Could you check a few things on this model? Use its own coordinates, in mm. Face numbers are marked on the shaded views. A direction names the side the tool comes from. Coordinates: 2 decimals unless noted, no trailing zeros. Order: outer loops, then holes, each group sorted by start corner. A loop starts at its lowest first (then second) coordinate and runs counter-clockwise, first axis right, second up.
```python
from build123d import *

# Parameters (mm, degrees)
SKETCH1_W                = 15
SKETCH1_H                = 20
SKETCH1_R                = 2.51
BOSS_EXTRUDE1_DEPTH      = 3
SKETCH2_R                = 4.51
CUT_EXTRUDE1_DEPTH       = 1
BOSS_EXTRUDE2_DEPTH      = 22
BOSS_EXTRUDE2_DEPTH_BACK = 3
SKETCH3_W                = 3
SKETCH3_H                = 20
SKETCH4_R                = 2.6
CUT_EXTRUDE2_DEPTH       = 22
BOSS_EXTRUDE3_START      = -3
SKETCH5_R                = 2.6
BOSS_EXTRUDE3_DEPTH      = 3
CUT_EXTRUDE3_DEPTH       = 5
SKETCH7_W                = 20
SKETCH7_H                = 20
BOSS_EXTRUDE4_DEPTH      = 3
SKETCH8_R                = 2.6
CUT_EXTRUDE6_DEPTH       = 3


with BuildPart() as part:
    # Sketch1 → Boss-Extrude1 (new body)
    with BuildSketch(Plane(origin=(0, 0, 0), x_dir=(1, 0, 0), z_dir=(0, 1, 0))):
        with Locations((23.125880705, 19.115097078)):
            Rectangle(SKETCH1_W, SKETCH1_H)
        with Locations(Location((23.125880705, 19.115097078, 0), (0, 0, 270))):
            Circle(SKETCH1_R, mode=Mode.SUBTRACT)
    extrude(amount=BOSS_EXTRUDE1_DEPTH)

    # Sketch2 → Cut-Extrude1 (cut)
    with BuildSketch(Plane(origin=(0, 3, 0), x_dir=(1, 0, 0), z_dir=(0, 1, 0))):
        with Locations(Location((23.125880705, 19.115097078, 0), (0, 0, 270))):
            Circle(SKETCH2_R)
    extrude(amount=-CUT_EXTRUDE1_DEPTH, mode=Mode.SUBTRACT)

    # Sketch3 → Boss-Extrude2 (add, two sides: drawn at the far end of the back side and taken through both)
    with BuildSketch(Plane(origin=(0, 3, 0), x_dir=(1, 0, 0), z_dir=(0, 1, 0)).offset(-BOSS_EXTRUDE2_DEPTH_BACK)):
        with Locations((14.125880705, 19.115097078)):
            Rectangle(SKETCH3_W, SKETCH3_H)
    extrude(amount=BOSS_EXTRUDE2_DEPTH + BOSS_EXTRUDE2_DEPTH_BACK)

    # Sketch4 → Cut-Extrude2 (cut)
    with BuildSketch(Plane.ZY.offset(-12.625880705)):
        with Locations((-23.115097078, 19)):
            Circle(SKETCH4_R)
        with Locations((-23.115097078, 6)):
            Circle(SKETCH4_R)
    extrude(amount=-CUT_EXTRUDE2_DEPTH, mode=Mode.SUBTRACT)

    # Sketch5 → Boss-Extrude3 (add)
    with BuildSketch(Plane(origin=(15.625880705, 0, 0), x_dir=(0, 0, -1), z_dir=(1, 0, 0)).offset(BOSS_EXTRUDE3_START)):
        with Locations((23.115097078, 19)):
            Circle(SKETCH5_R)
        with Locations((23.115097078, 6)):
            Circle(SKETCH5_R)
    extrude(amount=BOSS_EXTRUDE3_DEPTH)

    # Sketch6 → Cut-Extrude3 (cut)
    with BuildSketch(Plane(origin=(12.625880705, 25, -29.115097078), x_dir=(1, 0, 0), z_dir=(0, 1, 0))):
        Polygon((0, -14.855128206), (0, -20), (3, -20), (3, -14.855128206), (3, 0), (0, 0), align=None)
    extrude(amount=-CUT_EXTRUDE3_DEPTH, mode=Mode.SUBTRACT)

    # Sketch7 → Boss-Extrude4 (add)
    with BuildSketch(Plane.ZY.offset(-12.625880705)):
        with Locations((-19.115097078, 30)):
            Rectangle(SKETCH7_W, SKETCH7_H)
    extrude(amount=-BOSS_EXTRUDE4_DEPTH)

    # Sketch8 → Cut-Extrude6 (cut)
    with BuildSketch(Plane(origin=(15.625880705, 0, 0), x_dir=(0, 0, -1), z_dir=(1, 0, 0))):
        with Locations((13.915097078, 16)):
            Circle(SKETCH8_R)
        with Locations((13.915097078, 26.1)):
            Circle(SKETCH8_R)
    extrude(amount=-CUT_EXTRUDE6_DEPTH, mode=Mode.SUBTRACT)


solid = part.part
```
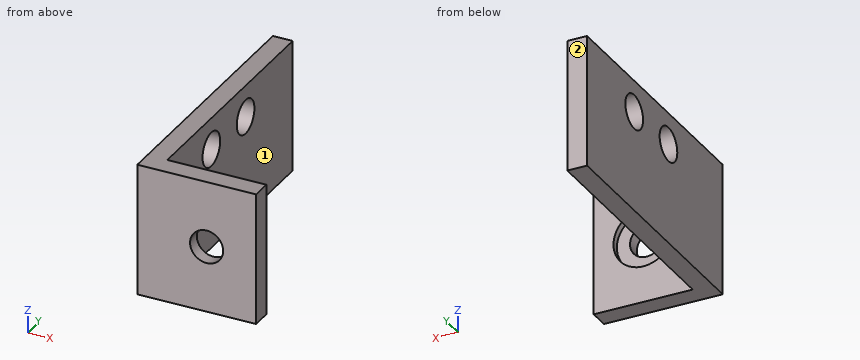
Item 1: I need wall thicknesses on line 1 (X direction, y = 11, z = -19); line 2 (Y direction, x = 21.75, z = -26); line 3 (Y direction, x = 24.5, z = -22.5). Which ranges of each line are inside material? Lowest first, please.
Item 2: Suppose I cut it at D-D (x = 22.25). List the corners of the cut face in (y, z) for me.
Item 3: Suppose I cut it at C-C (z = -13). List the corners of the cut face in (x, y) for me, and give its area (3 significant figures).
Item 4: For pin 1 Ø1 at (y, z) = (32.5, -17.5) entering from +X; pin 2 Ø4.5 at (y, z) = (16, -13.92) entering from -X; pin 3 Ø2 at (x, z) = (20, -14) entering from -Y; pin 4 Ø1 at (x, z) = (21, -19.5) entering from +Y, each with a flat end and sliding along its axis, tell me the tip position at first contact or that it passes through.
Item 5: Which directions (+Z, -Z, +X, -X, +Y, -Y) give clear straight access to the entire face, cutting with the end or side of a thin tool? Please do the marked faces 1 and 2.
Item 6: Suppose I cut it at A-A (y = 26.1). List the corners of the cut face in (x, z) for me.
Item 7: Suppose I cut it at B-B (x = 14.75). List the corners of the cut face in (y, z) for me, and give its area (3 significant figures).
Geometry results:
1. line 1: x = 12.63 to 15.63
1. line 2: y = 0 to 3
1. line 3: y = 0 to 2
2. outline: (0, -29.12) - (3, -29.12) - (3, -23.54) - (2, -23.54) - (2, -21.47) - (0, -21.47) - close; (0, -16.76) - (2, -16.76) - (2, -14.69) - (3, -14.69) - (3, -9.12) - (0, -9.12) - close
3. outline: (12.63, 0) - (30.63, 0) - (30.63, 3) - (15.63, 3) - (15.63, 13.57) - (12.63, 13.57) - close; (12.63, 18.43) - (15.63, 18.43) - (15.63, 23.67) - (12.63, 23.67) - close; (12.63, 28.53) - (15.63, 28.53) - (15.63, 40) - (12.63, 40) - close
3. area: 136 mm2
4. pin 1: stops at x = 15.63
4. pin 2: passes through
4. pin 3: stops at y = 0
4. pin 4: stops at y = 2
5. face 1: +Z, -Z, +X, +Y
5. face 2: +Z, -Z, +X, -X, +Y
6. outline: (12.63, -29.12) - (15.63, -29.12) - (15.63, -16.52) - (12.63, -16.52) - close; (12.63, -11.32) - (15.63, -11.32) - (15.63, -9.12) - (12.63, -9.12) - close
7. outline: (0, -29.12) - (40, -29.12) - (40, -9.12) - (0, -9.12) - close; hole circle Ø5.2 at (16, -13.92); hole circle Ø5.2 at (26.1, -13.92)
7. area: 758 mm2
